Source: CAD feature listing. Evaluate the final solid. Frame: model axes, mm. Give positions to 0.01 mm unless a question says otherwise; leave off trailing zeros. Order: outer loops, then holes, each group sorted by start corner. A loop starts at its lowest first (then second) coordinate and runs counter-clockwise, first axis right, second up. Notation, with made-up numbers: (88.25, 9) - (92.25, 9) arc R12 ccw to (92.25, 20) - close; hole circle Ø6 at (-33.5, -13.75). An arc over 180 degrees is marked (long way). Write each question's results on one line, items separated by ' | '. Start each with the question number.
Item 1: Section B-B on z = 0.9. State how many separate pieces and enclosed holes the cut face has, and give its area (3 significant figures).
Item 2: Mould query, pull axis Y, two halves, no side actions, for faces 1 (the cylindrical face through (-28, -21, 2)), 2 (the flat face through (102, 1, 0)), 3 (the cylindrical face through (259.985, 1.319, 1.972)). Classes: released by +Y, released by -Y, zero draft, split by the parting line, or undercut.
Item 3: Contact query for flat-ended pins moving along their axis: pin 1 Ø4 at (x, y) = (-44.25, 0) entering from -Z; pin 2 Ø1.5 at (y, z) = (-15, 3.5) entering from +X; pin 3 Ø3.5 at (x, y) = (-31.29, -31.29) entering from +Z; pin 4 Ø1 at (y, z) = (-31, 2.5) entering from -X. Output: stop coordinate, or through.
Item 4: Line query: line 1 along Y through (x, z) = (0, 2.1); line 2 along Y through (x, z) = (-32, 1.4); line 3 along X through (y, z) = (-28, 1). Output: solid intervals per line, ascending.
Item 5: Section A-A on y = 8.5. Output: boundary loops of the cut face in (x, z), and give its area (3 significant figures).
Item 6: Section C-C on x = 218. Output: boundary loops of the cut face in (y, z), and give its area (3 significant figures).
Item 7: Section D-D on y = 22. Output: boundary loops of the cut face in (x, z).
```python
from build123d import *

# Parameters (mm, degrees)
SKETCH_1_R          = 35
EXTRUDE_1_DEPTH     = 4
SKETCH_2_R          = 1.6
CUT_EXTRUDE_1_DEPTH = 5
CHAMFER_1_SIZE      = 1


with BuildPart() as part:
    # 草图1 → 凸台-拉伸1 (new body)
    with BuildSketch(Plane.XY):
        with BuildLine():
            Line((0, 60), (200, 60))
            ThreePointArc((200, 60), (260, 0), (200, -60))
            Line((200, -60), (0, -60))
            ThreePointArc((0, -60), (-60, 0), (0, 60))
        make_face()
        Circle(SKETCH_1_R, mode=Mode.SUBTRACT)
        with Locations((200, 0)):
            Circle(SKETCH_1_R, mode=Mode.SUBTRACT)
    extrude(amount=EXTRUDE_1_DEPTH)

    # 草图2 → 切除-拉伸1 (cut)
    with BuildSketch(Plane.XY.offset(4)):
        with Locations((0, 42.5)):
            Circle(SKETCH_2_R)
        with Locations((0, -42.5)):
            Circle(SKETCH_2_R)
        with Locations((44.25, 0)):
            Circle(SKETCH_2_R)
        with Locations((31.289475068, -31.289475068)):
            Circle(SKETCH_2_R)
        with Locations((-31.289475068, -31.289475068)):
            Circle(SKETCH_2_R)
        with Locations((-44.25, 0)):
            Circle(SKETCH_2_R)
        with Locations((-31.289475068, 31.289475068)):
            Circle(SKETCH_2_R)
        with Locations((31.289475068, 31.289475068)):
            Circle(SKETCH_2_R)
        with Locations((168.710524932, -31.289475068)):
            Circle(SKETCH_2_R)
        with Locations((231.289475068, -31.289475068)):
            Circle(SKETCH_2_R)
        with Locations((200, -42.5)):
            Circle(SKETCH_2_R)
        with Locations((155.75, 0)):
            Circle(SKETCH_2_R)
        with Locations((244.25, 0)):
            Circle(SKETCH_2_R)
        with Locations((168.710524932, 31.289475068)):
            Circle(SKETCH_2_R)
        with Locations((200, 42.5)):
            Circle(SKETCH_2_R)
        with Locations((231.289475068, 31.289475068)):
            Circle(SKETCH_2_R)
    extrude(amount=-CUT_EXTRUDE_1_DEPTH, mode=Mode.SUBTRACT)

    # 倒角1
    chamfer_1_edges = [part.edges().sort_by_distance(p)[0] for p in [
        (-45.85, 0, 4),
        (-32.889475068, -31.289475068, 4),
        (29.689475068, 31.289475068, 4),
        (-1.6, 42.5, 4),
        (167.110524932, 31.289475068, 4),
        (154.15, 0, 4),
        (167.110524932, -31.289475068, 4),
        (198.4, -42.5, 4),
        (229.689475068, -31.289475068, 4),
        (242.65, 0, 4),
        (229.689475068, 31.289475068, 4),
        (198.4, 42.5, 4),
        (-1.6, -42.5, 4),
        (29.689475068, -31.289475068, 4),
        (42.65, 0, 4),
        (-32.889475068, 31.289475068, 4),
    ]]
    chamfer(chamfer_1_edges, length=CHAMFER_1_SIZE)


solid = part.part
```
Evaluation:
1) separate pieces: 1 | enclosed holes: 18 | area: 27,500 mm^2
2) face 1: undercut | face 2: zero draft | face 3: split by the parting line
3) pin 1: stops at z = 0 | pin 2: stops at x = 258.28 | pin 3: stops at z = 3.15 | pin 4: stops at x = -51.67
4) line 1: y = -60 to -44.1, -40.9 to -35, 35 to 40.9, 44.1 to 60 | line 2: y = -50.75 to -32.72, -29.86 to -14.18, 14.18 to 29.86, 32.72 to 50.75 | line 3: x = -53.07 to -21, 21 to 179, 221 to 253.07
5) outline: (-59.39, 0) - (-33.95, 0) - (-33.95, 4) - (-59.39, 4) - close; (33.95, 0) - (166.05, 0) - (166.05, 4) - (33.95, 4) - close; (233.95, 0) - (259.39, 0) - (259.39, 4) - (233.95, 4) - close | area: 732 mm^2
6) outline: (-57.24, 0) - (-30.02, 0) - (-30.02, 4) - (-57.24, 4) - close; (30.02, 0) - (57.24, 0) - (57.24, 4) - (30.02, 4) - close | area: 218 mm^2
7) outline: (-55.82, 0) - (-27.22, 0) - (-27.22, 4) - (-55.82, 4) - close; (27.22, 0) - (172.78, 0) - (172.78, 4) - (27.22, 4) - close; (227.22, 0) - (255.82, 0) - (255.82, 4) - (227.22, 4) - close
